The listing builds one solid part. Answer for the finished solid, in the listing's coordinates (mm). Coordinates: 2 decimals unless noted, no trailing zeros. Order: outer loops, then holes, each group sorted by start corner. A loop starts at its lowest first (then second) coordinate and runs counter-clockwise, first axis right, second up. Notation, with made-up numbers: (-8.75, 2) - (47.25, 2) arc R16 ccw to (47.25, 6) - close; hole circle Ø2 at (62, 28.5). An arc over 180 degrees is marked (long way). Use one line per item in the form item = value. Start each with the question number.
Item 1: Section A-A, the plane z = -43 is taken. Write down the section's boundary in (x, y), and give its area (3 significant figures).
Item 2: Each of these flat-tipped pins is pushed along its axis until it touches: pin 1 Ø1.6 at (x, z) = (150, -53) entering from -Y; pin 2 Ø1.7 at (y, z) = (3, -38.5) entering from -X; pin 3 Ø3 at (y, z) = (4, -32) entering from +X. Where does it stop, or does it pass through?
Item 3: Section C-C, the plane y = 3.4 is taken. Count the separate pieces of the cut face and the enclosed holes in it, and give its area (3 significant figures).
Item 4: Section B-B, the plane x = 141 is taken. Write down the section's boundary in (y, z), and give its area (4 significant figures).
Item 5: Consider line 1 along X through (y, z) = (1.5, -90); line 2 along X through (y, z) = (3.45, -53); line 3 along Z through (x, y) = (90, 1.35). Determine where each line is inside the solid, lowest interval first. Write a range as [from, to].
from build123d import *

# Parameters (mm, degrees)
SKETCH3_W           = 192
SKETCH3_H           = 135
BOSS_EXTRUDE1_DEPTH = 5.7
SKETCH9_W           = 115
SKETCH9_H           = 70
CUT_EXTRUDE2_DEPTH  = 47
SKETCH12_R          = 1
CUT_EXTRUDE3_DEPTH  = 37
CUT_EXTRUDE4_DEPTH  = 11


with BuildPart() as part:
    # Sketch3 → Boss-Extrude1 (new body)
    with BuildSketch(Plane(origin=(0, 0, 0), x_dir=(1, 0, 0), z_dir=(0, 1, 0))):
        with Locations((90, 53.5)):
            Rectangle(SKETCH3_W, SKETCH3_H)
    extrude(amount=BOSS_EXTRUDE1_DEPTH)

    # Sketch9 → Cut-Extrude2 (cut)
    with BuildSketch(Plane(origin=(0, 0, 0), x_dir=(1, 0, 0), z_dir=(0, 1, 0))):
        with Locations((90, 53)):
            Rectangle(SKETCH9_W, SKETCH9_H)
    extrude(amount=CUT_EXTRUDE2_DEPTH, mode=Mode.SUBTRACT)

    # Sketch12 → Cut-Extrude3 (cut)
    with BuildSketch(Plane(origin=(0, 0, 0), x_dir=(1, 0, 0), z_dir=(0, 1, 0))):
        with Locations((30, 90)):
            Circle(SKETCH12_R)
        with Locations((30, 53)):
            Circle(SKETCH12_R)
        with Locations((30, 16)):
            Circle(SKETCH12_R)
        with Locations((90, 16)):
            Circle(SKETCH12_R)
        with Locations((150, 16)):
            Circle(SKETCH12_R)
        with Locations((150, 53)):
            Circle(SKETCH12_R)
        with Locations((150, 90)):
            Circle(SKETCH12_R)
        with Locations((90, 90)):
            Circle(SKETCH12_R)
    extrude(amount=CUT_EXTRUDE3_DEPTH, mode=Mode.SUBTRACT)

    # Sketch13 → Cut-Extrude4 (cut)
    with BuildSketch(Plane(origin=(0, 0, 0), x_dir=(1, 0, 0), z_dir=(0, 1, 0))):
        Polygon((-5.7, 121), (-5.7, 94), (0, 94), (0, 67), (-5.7, 67), (-5.7, 40), (0, 40), (0, 13), (-5.7, 13), (-5.7, -14), (-9.7, -14), (-9.7, 121), align=None)
        Polygon((189.7, 121), (185.7, 121), (185.7, 94), (180, 94), (180, 67), (185.7, 67), (185.7, 40), (180, 40), (180, 13), (185.7, 13), (185.7, -14), (189.7, -14), align=None)
    extrude(amount=CUT_EXTRUDE4_DEPTH, mode=Mode.SUBTRACT)


solid = part.part
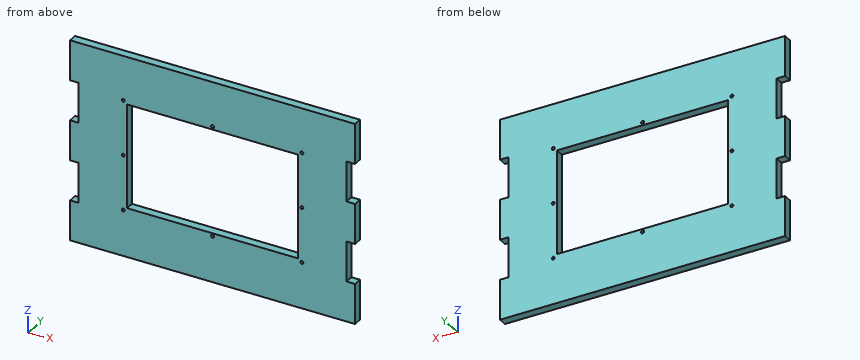
Response:
q1.outline = (-5.7, 0) - (32.5, 0) - (32.5, 5.7) - (-5.7, 5.7) - close; (147.5, 0) - (185.7, 0) - (185.7, 5.7) - (147.5, 5.7) - close
q1.area = 435 mm2
q2.pin_1 = through
q2.pin_2 = 0
q2.pin_3 = 180
q3.separate_pieces = 1
q3.enclosed_holes = 9
q3.area = 17,100 mm2
q4.outline = (0, -121) - (5.7, -121) - (5.7, -88) - (0, -88) - close; (0, -18) - (5.7, -18) - (5.7, 14) - (0, 14) - close
q4.area = 370.5 mm2
q5.line_1 = [0, 29], [31, 89], [91, 149], [151, 180]
q5.line_2 = [-5.7, 29], [31, 32.5], [147.5, 149], [151, 185.7]
q5.line_3 = [-121, -91], [-89, -88], [-18, -17], [-15, 14]
